Geometry check sheet. Reference: the model listing, model coordinates, mm. Face numbers are marked on the shaded views. A direction names the side the tool comes from. Give positions to 0.01 mm unless a question says otherwise; leave off trailing zeros. Order: outer loops, then holes, each group sorted by start corner. A loop starts at its lowest first (then second) coordinate and runs counter-clockwise, first axis right, second up.
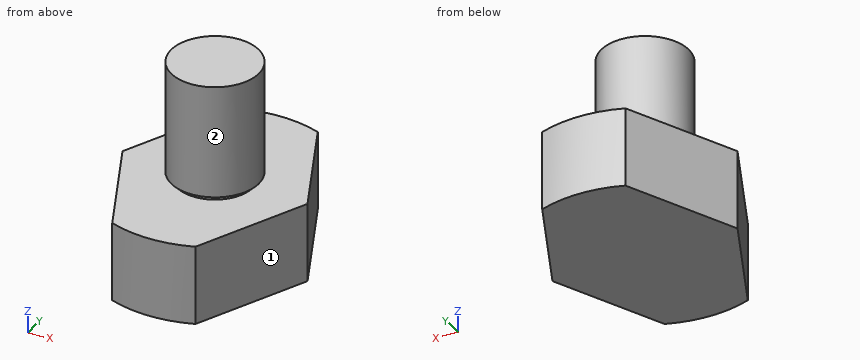
from build123d import *

# Parameters (mm, degrees)
CUT_EXTRUDE_START   = -30
SKETCH_2_R          = 36.239320701
CUT_EXTRUDE_1_DEPTH = 30


with BuildPart() as part:
    # 草图1 → 旋转1 (revolve)
    with BuildSketch(Plane(origin=(0, 0, 0), x_dir=(1, 0, 0), z_dir=(0, 1, 0))):
        Polygon((0, 0), (0, 50), (30, 50), (30, 30), (9.5, 30), (9.5, 28.5), (11, 28.5), (11, 0), align=None)
    revolve(axis=Axis((0, 0, 0), (0, 0, -1)))

    # 草图2 → 切除-拉伸1 (cut)
    with BuildSketch(Plane(origin=(0, 0, -50), x_dir=(-1, 0, 0), z_dir=(0, 0, -1)).offset(CUT_EXTRUDE_START)):
        Circle(SKETCH_2_R)
        with BuildLine():
            Line((-10.527630828, 28.092151736), (-23.409516673, 0))
            Line((-23.409516673, 0), (-10.527630828, -28.092151736))
            ThreePointArc((-10.527630828, -28.092151736), (0, -30), (10.527630828, -28.092151736))
            Line((10.527630828, -28.092151736), (23.409516673, 0))
            Line((23.409516673, 0), (10.527630828, 28.092151736))
            ThreePointArc((10.527630828, 28.092151736), (0, 30), (-10.527630828, 28.092151736))
        make_face(mode=Mode.SUBTRACT)
    extrude(amount=CUT_EXTRUDE_1_DEPTH, mode=Mode.SUBTRACT)


solid = part.part
Item 1: Gauge pin test, flat ends, axial feed: pin 1 (8 mm diameter, centred on y = 17, z = -23.5, fed in from +X); pin 2 (2 mm diameter, centred on x = 9, z = -38, fed in from +Y); pin 3 (10 mm diameter, centred on x = 10.5, z = -13.5, fed in from -Y); pin 4 (12 mm diameter, centred on x = -17, y = 13.5, fed in from +Z). Record the tip position at first contact, or that the pin passes through.
Reported:
pin 1: passes through
pin 2: stops at y = 28.91
pin 3: stops at y = -9.53
pin 4: stops at z = -30
Item 2: Sectioned sample at B-B (z = -33). Enter the section's corners in (x, y), and give its area (3 significant figures).
Reported:
outline: (-23.41, 0) - (-10.53, -28.09) arc R30 ccw to (10.53, -28.09) - (23.41, 0) - (10.53, 28.09) arc R30 ccw to (-10.53, 28.09) - close
area: 1,960 mm2
Item 3: Sectioned sample at C-C (y = -3.5). Enter the section's corners in (x, z), and give its area (3 significant figures).
Reported:
outline: (-21.8, -50) - (21.8, -50) - (21.8, -30) - (8.83, -30) - (8.83, -28.5) - (10.43, -28.5) - (10.43, 0) - (-10.43, 0) - (-10.43, -28.5) - (-8.83, -28.5) - (-8.83, -30) - (-21.8, -30) - close
area: 1,490 mm2
Item 4: Sectioned sample at A-A (x = 0). Enter the section's corners in (y, z), and give its area (3 significant figures).
Reported:
outline: (-30, -50) - (30, -50) - (30, -30) - (9.5, -30) - (9.5, -28.5) - (11, -28.5) - (11, 0) - (-11, 0) - (-11, -28.5) - (-9.5, -28.5) - (-9.5, -30) - (-30, -30) - close
area: 1,860 mm2
Item 5: Sectioned sample at D-D (z = -26.5). Enter the section's corners in (x, y).
Reported:
outline: circle Ø22 at (0, 0)
Item 6: Scan lines: L1, parallel to Z at x = 1, y = 10.5; L2, parallel to Z at x = 16, y = 7; L3, parallel to X at y = 0, z = -7.5. Record each from-to range of solid material in increasing order.
Reported:
L1: z = -50 to -30, -28.5 to 0
L2: z = -50 to -30
L3: x = -11 to 11
Item 7: Set-up check for the marked faces 1 and 2: record each of +Z, -Z, +X, -X, +Y, -Y from which the full face is reachable in a straight line by a thin tool's end or side.
Reported:
face 1: +Z, -Z, +X, -Y
face 2: +Z
